```python
from build123d import *

# Parameters (mm, degrees)
BOSS_EXTRUDE1_DEPTH = 25.4
CIRPATTERN1_COUNT   = 6


with BuildPart() as part:
    # Sketch1 → Boss-Extrude1 (new body)
    with BuildSketch(Plane(origin=(0, 0, 0), x_dir=(1, 0, 0), z_dir=(0, 1, 0))):
        Polygon((25.4, 0), (12.7, 21.997045256), (-12.7, 21.997045256), (-25.4, 0), (-12.7, -21.997045256), (12.7, -21.997045256), align=None)
    extrude(amount=BOSS_EXTRUDE1_DEPTH)

    # Sketch2 → 1/4 NPT Tapped Hole1 (revolve, cut)
    with BuildSketch(Plane(origin=(0, 0, 0), x_dir=(0, 0, -1), z_dir=(1, 0, 0))):
        Polygon((0, 0), (0, 20.360347279), (5.5626, 17.018), (5.5626, 9.906), (6.557984794, 9.906), (6.8545837, 0), align=None)
    revolve(axis=Axis((0, -6.35, 0), (0, 1, 0)), mode=Mode.SUBTRACT)

    # Sketch4 → 1/4 NPT Tapped Hole2 (revolve, cut)
    with BuildSketch(Plane(origin=(0, 12.7, 21.997045256), x_dir=(0, -1, 0), z_dir=(1, 0, 0))):
        Polygon((0, 0), (0, 20.360347279), (5.5626, 17.018), (5.5626, 9.906), (6.557984794, 9.906), (6.8545837, 0), align=None)
    f_1_4_npt_tapped_hole2 = revolve(axis=Axis((0, 12.7, 28.347045256), (0, 0, -1)), mode=Mode.SUBTRACT)

    # CirPattern1: 1/4 NPT Tapped Hole2 ×6 about axis
    cirpattern1_axis = Axis((0, 0, 0), (0, 1, 0))
    for i in range(1, CIRPATTERN1_COUNT):
        add(f_1_4_npt_tapped_hole2.rotate(cirpattern1_axis, i * 360 / CIRPATTERN1_COUNT), mode=Mode.SUBTRACT)


solid = part.part
```
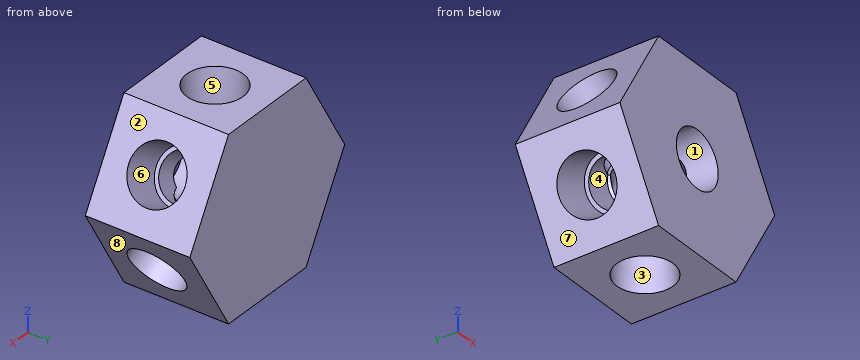
The model under review builds one solid part; all positions refer to its coordinate system, in mm. Face numbers are marked on the shaded views. A direction names the side the tool comes from. Coordinates: 2 decimals unless noted, no trailing zeros. Write each loop counter-clockwise with the first axis right and the second up, starting at its lowest first coordinate (ties: lowest second). Pieces come first, ordered by that corner, then holes. Notation, with made-up numbers: (79, 14) - (89, 14) arc R14 cw to (89, 39) - close; hole circle Ø1 at (78.5, 55.25). An arc over 180 degrees is marked (long way). Answer in a Markdown table with one row per item. Add a question column.
Q1. Consider section B-B on x = -1.5. Give the number of separate pieces and of enclosed holes in the cut face, then the cut area to 3 significant figures.
Q2. To check wall thickness, follow line 1 along Z through (x, y) = (-8, 11.5); line 2 along Y through (x, z) = (0, 7.5); line 3 along Z through (x, y) = (-13.5, 13). State the ranges of each line that lie inside material, in increasing order. Write a range as from..to.
Q3. Clearance check with flat-ended pins moving along their axes: pin 1 (10 mm diameter, centred on x = 0, y = 12.7, fed in from +Z); pin 2 (8 mm diameter, centred on y = 18, z = -12, fed in from +X); pin 3 (1.5 mm diameter, centred on y = 16, z = 13, fed in from +X). State where each tip first meets the part, or that it passes through.
Q4. Consider section C-C on z = 19. Give the boundary of the cut face in (x, y).
Q5. Draft analysis for pull direction X (two halves, no side actions). For the marked faces 6, 7 and 8, state which applies: +X half, -X half, draft (parallel to the pull), parting line (faces both ways), or undercut.
Q6. Consider section A-A on y = 22.75. Give the boundary of the cut face in (x, z), then the cut area to 3 significant figures.
Q7. For the marked faces 1, 2, 3, 4 and 5, list the 3-axis set-ups (+Z, -Z, +X, -X, +Y, -Y) from which the entire face can be reached by the end or side of a thin tool; tool diameter is ignored.
Answers below:
| question | item | result |
|---|---|---|
| 1 | separate pieces | 3 |
| 1 | enclosed holes | 0 |
| 1 | area | 498 mm² |
| 2 | line 1 | -22..-12.09, 12.09..22 |
| 2 | line 2 | 0..7.14, 18.26..25.4 |
| 2 | line 3 | -20.61..-15.62, -0.8..0.8, 15.62..20.61 |
| 3 | pin 1 | z = 4.64 |
| 3 | pin 2 | x = 20.75 |
| 3 | pin 3 | x = 12.4 |
| 4 | outline | (-14.43, 0) - (14.43, 0) - (14.43, 25.4) - (-14.43, 25.4) - close; hole circle Ø13.53 at (0, 12.7) |
| 5 | face 6 | undercut |
| 5 | face 7 | -X half |
| 5 | face 8 | +X half |
| 6 | outline | (-25.4, 0) - (-12.7, -22) - (12.7, -22) - (25.4, 0) - (12.7, 22) - (-12.7, 22) - close |
| 6 | area | 1,680 mm² |
| 7 | face 1 | -Y |
| 7 | face 2 | +Z, +X, +Y, -Y |
| 7 | face 3 | -Z |
| 7 | face 4 | none |
| 7 | face 5 | +Z |
